Design review of the part built by this model. Coordinates are the model's own, in mm. A direction names the side the tool comes from. Give positions to 0.01 mm unless a question says otherwise; leave off trailing zeros. Order: outer loops, then holes, each group sorted by start corner. A loop starts at its lowest first (then second) coordinate and runs counter-clockwise, first axis right, second up. Notation, with made-up numbers: (9, 44.5) -> (23, 44.5) arc R28 ccw to (23, 80.5) -> close; hole circle Ø10 at (20, 77.5). An arc over 180 degrees is marked (long way). Answer in a Markdown table with one row per item. Add a question column.
```python
from build123d import *

# Parameters (mm, degrees)
CROQUIS1_W                = 13
CROQUIS1_H                = 80
SALIENTE_EXTRUIR1_DEPTH   = 4
CROQUIS1_W_2              = 10
SALIENTE_EXTRUIR1_2_DEPTH = 4
SALIENTE_EXTRUIR1_3_DEPTH = 4
CROQUIS2_W                = 13
CROQUIS2_H                = 13
CROQUIS2_W_2              = 10
CROQUIS2_H_2              = 10
SALIENTE_EXTRUIR2_DEPTH   = 10
CROQUIS3_W                = 13
CROQUIS3_H                = 80
CROQUIS3_W_2              = 10
SALIENTE_EXTRUIR3_DEPTH   = 2.2
CROQUIS4_W                = 80
CROQUIS4_H                = 10
CROQUIS4_H_2              = 13
SALIENTE_EXTRUIR4_DEPTH   = 4
CROQUIS5_W                = 80
CROQUIS5_H                = 80
CROQUIS5_W_2              = 75.6
CROQUIS5_H_2              = 75.6
SALIENTE_EXTRUIR5_DEPTH   = 15
CHAFL_N2_SIZE             = 6.4
CHAFL_N3_SIZE             = 6
CHAFL_N4_SIZE             = 2.2
CROQUIS6_W                = 10
CROQUIS6_H                = 10
CORTAR_EXTRUIR1_DEPTH     = 0.4
REDONDEO1_R               = 1
CHAFL_N1_SIZE             = 1


with BuildPart() as part:
    # Croquis1 → Saliente-Extruir1 (new body)
    with BuildSketch(Plane(origin=(0, 0, 0), x_dir=(0, 1, 0), z_dir=(0, 0, 1))):
        Rectangle(CROQUIS1_W, CROQUIS1_H)
    extrude(amount=SALIENTE_EXTRUIR1_DEPTH)



with BuildPart() as body_2:
    # Croquis1 → Saliente-Extruir1 2 (new body)
    with BuildSketch(Plane(origin=(0, 0, 0), x_dir=(0, 1, 0), z_dir=(0, 0, 1))):
        with Locations((35, 0)):
            Rectangle(CROQUIS1_W_2, CROQUIS1_H)
    extrude(amount=SALIENTE_EXTRUIR1_2_DEPTH)


with BuildPart() as body_3:
    # Croquis1 → Saliente-Extruir1 3 (new body)
    with BuildSketch(Plane(origin=(0, 0, 0), x_dir=(0, 1, 0), z_dir=(0, 0, 1))):
        with Locations((-35, 0)):
            Rectangle(CROQUIS1_W_2, CROQUIS1_H)
    extrude(amount=SALIENTE_EXTRUIR1_3_DEPTH)


with BuildPart() as part_1:
    add(part.part)

    add(body_2.part)  # Saliente-Extruir2 merges body 2

    add(body_3.part)  # Saliente-Extruir2 merges body 3
    # Croquis2 → Saliente-Extruir2 (add)
    with BuildSketch(Plane.XY.offset(4)):
        Rectangle(CROQUIS2_W, CROQUIS2_H)
        with Locations((-35, 0)):
            Rectangle(CROQUIS2_W_2, CROQUIS2_H)
        with Locations((35, 0)):
            Rectangle(CROQUIS2_W_2, CROQUIS2_H)
        with Locations((0, 35)):
            Rectangle(CROQUIS2_W, CROQUIS2_H_2)
        with Locations((-35, 35)):
            Rectangle(CROQUIS2_W_2, CROQUIS2_H_2)
        with Locations((35, 35)):
            Rectangle(CROQUIS2_W_2, CROQUIS2_H_2)
        with Locations((35, -35)):
            Rectangle(CROQUIS2_W_2, CROQUIS2_H_2)
        with Locations((-35, -35)):
            Rectangle(CROQUIS2_W_2, CROQUIS2_H_2)
        with Locations((0, -35)):
            Rectangle(CROQUIS2_W, CROQUIS2_H_2)
    extrude(amount=SALIENTE_EXTRUIR2_DEPTH)

    # Croquis3 → Saliente-Extruir3 (add)
    with BuildSketch(Plane.XY.offset(14)):
        Rectangle(CROQUIS3_W, CROQUIS3_H)
        with Locations((-35, 0)):
            Rectangle(CROQUIS3_W_2, CROQUIS3_H)
        with Locations((35, 0)):
            Rectangle(CROQUIS3_W_2, CROQUIS3_H)
    extrude(amount=-SALIENTE_EXTRUIR3_DEPTH)

    # Croquis4 → Saliente-Extruir4 (add)
    with BuildSketch(Plane.XY.offset(14)):
        with Locations((0, -35)):
            Rectangle(CROQUIS4_W, CROQUIS4_H)
        Rectangle(CROQUIS4_W, CROQUIS4_H_2)
        with Locations((0, 35)):
            Rectangle(CROQUIS4_W, CROQUIS4_H)
        with Locations((0, 16.5)):
            Rectangle(CROQUIS4_W, CROQUIS4_H)
        with Locations((0, -16.5)):
            Rectangle(CROQUIS4_W, CROQUIS4_H)
    extrude(amount=SALIENTE_EXTRUIR4_DEPTH)

    # Croquis5 → Saliente-Extruir5 (add)
    with BuildSketch(Plane.XY.offset(14)):
        Rectangle(CROQUIS5_W, CROQUIS5_H)
        Rectangle(CROQUIS5_W_2, CROQUIS5_H_2, mode=Mode.SUBTRACT)
    extrude(amount=SALIENTE_EXTRUIR5_DEPTH)

    # Chaflán2
    chafl_n2_edges = [part_1.edges().sort_by_distance(p)[0] for p in [
        (0, -30, 11.8),
        (-35, 6.5, 11.8),
        (-35, -6.5, 11.8),
        (-35, 30, 11.8),
        (-35, -30, 11.8),
        (35, 6.5, 11.8),
        (35, 30, 11.8),
        (35, -6.5, 11.8),
        (35, -30, 11.8),
        (0, 6.5, 11.8),
        (0, -6.5, 11.8),
        (0, 30, 11.8),
    ]]
    chamfer(chafl_n2_edges, length=CHAFL_N2_SIZE)

    # Chaflán3
    chafl_n3_edges = [part_1.edges().sort_by_distance(p)[0] for p in [
        (-6.5, -35, 14),
        (30, -35, 14),
        (6.5, 35, 14),
        (-30, 35, 14),
        (6.5, -35, 14),
        (-6.5, 35, 14),
        (-30, -35, 14),
        (30, 35, 14),
    ]]
    chamfer(chafl_n3_edges, length=CHAFL_N3_SIZE)

    # Chaflán4
    chafl_n4_edges = [part_1.edges().sort_by_distance(p)[0] for p in [
        (30, 16.5, 14),
        (30, -16.5, 14),
        (6.5, -16.5, 14),
        (-6.5, -16.5, 14),
        (-30, -16.5, 14),
        (6.5, 16.5, 14),
        (-30, 16.5, 14),
    ]]
    chamfer(chafl_n4_edges, length=CHAFL_N4_SIZE - 0.0001)  # a hair under: the kernel refuses the full size

    # Croquis6 → Cortar-Extruir1 (cut)
    with BuildSketch(Plane(origin=(-40, 0, 0), x_dir=(0, -1, 0), z_dir=(-1, 0, 0))):
        with Locations((0, 14.5)):
            Rectangle(CROQUIS6_W, CROQUIS6_H)
    extrude(amount=-CORTAR_EXTRUIR1_DEPTH, mode=Mode.SUBTRACT)

    # Redondeo1
    redondeo1_edges = [part_1.edges().sort_by_distance(p)[0] for p in [
        (-39.8, -5, 19.5),
        (-39.8, -5, 9.5),
        (-39.8, 5, 9.5),
        (-39.8, 5, 19.5),
    ]]
    fillet(redondeo1_edges, radius=REDONDEO1_R)

    # Chaflán1
    chafl_n1_edges = [part_1.edges().sort_by_distance(p)[0] for p in [
        (-40, 40, 14.5),
        (-40, -40, 14.5),
        (40, -40, 14.5),
        (40, 6.5, 2.7),
        (-40, 6.5, 2.7),
        (-30, 6.5, 4.7),
        (-6.5, 6.5, 4.7),
        (6.5, 6.5, 4.7),
        (30, 6.5, 4.7),
        (6.5, -6.5, 4.7),
        (-30, -6.5, 4.7),
        (-40, -6.5, 2.7),
        (40, -6.5, 2.7),
        (-40, -18.25, 11.8),
        (30, 30, 4.7),
        (-6.5, 30, 4.7),
        (-30, 30, 4.7),
        (-40, 30, 2.7),
        (40, 30, 2.7),
        (-40, 18.25, 11.8),
        (40, -30, 2.7),
        (-40, -30, 2.7),
        (-30, -30, 4.7),
        (6.5, -30, 4.7),
        (30, -30, 4.7),
        (40, 18.25, 11.8),
        (40, -18.25, 11.8),
        (-40, -9.7, 8.6),
        (-40, 26.8, 8.6),
        (-40, 9.7, 8.6),
        (-40, -26.8, 8.6),
        (40, 9.7, 8.6),
        (40, 26.8, 8.6),
        (40, -9.7, 8.6),
        (40, -26.8, 8.6),
        (30, 40, 6),
        (30, -40, 6),
        (-30, 40, 6),
        (-30, -40, 6),
        (6.5, 40, 6),
        (-6.5, -40, 6),
        (6.5, -40, 6),
        (-6.5, 40, 6),
        (40, 40, 14.5),
    ]]
    chamfer(chafl_n1_edges, length=CHAFL_N1_SIZE)


solid = part_1.part
```
1) Add section B-B, the plane z = 22. Write out the cut boundary in (x, y), and give its area (3 significant figures).
2) Clearance check with flat-ended pins moving along their axes: P1, Ø4, axis at x = -5, y = -27.5, coming from the +Z side; P2, Ø8, axis at x = -22, y = 33.5, coming from the +Z side; P3, Ø10, axis at y = 12, z = 11.5, coming from the -X side; P4, Ø8, axis at x = -1.5, y = -16.5, coming from the -Z side. State where each tip first meets the part, or that it passes through.
3) Add section C-C, the plane y = 26. Write out the cut boundary in (x, z), and give its area (3 significant figures).
4) For L1, parallel to X at y = 5.5, z = 11.25; L2, parallel to Y at x = 12, z = 14.5, list the stretches that pass through material, from the lowest coordinate up.
5) Machinability: for faces 4 (the face through (-1, -30, 2)), 5 (the face through (18, 0, 14)), 6 (the face through (39.493, 27.1, 8.998)), 7 (the face through (18, 17, 14)), 8 (the face through (-1, -6.5, 16)), which of the approach directions +Z, -Z, +X, -X, +Y, -Y give a long, thin tool a straight path to every point of the face, cutting with its end or side? Answer none if there is none.
6) Add section A-A, the plane z = 2.5. Write out the cut boundary in (x, y), and give its area (3 significant figures).
7) Mouldability with a two-part tool opening along X and no side actions: class faces 1 (the face through (-35, -18, 11.8)), 2 (the face through (-18, 35, 14)), 3 (the face through (39.493, -27.1, 8.998)) as +X half, -X half, draft (parallel to the pull), parting line (faces both ways), or undercut.
8) Add section D-D, the plane y = -1.5. Write out the cut boundary in (x, z).
Verdict:
| question | item | result |
|---|---|---|
| 1 | outline | (-40, -39) -> (-39, -40) -> (39, -40) -> (40, -39) -> (40, 39) -> (39, 40) -> (-39, 40) -> (-40, 39) -> close; hole (-37.8, -37.8) -> (37.8, -37.8) -> (37.8, 37.8) -> (-37.8, 37.8) -> close |
| 1 | area | 683 mm2 |
| 2 | P1 | stops at z = 14 |
| 2 | P2 | stops at z = 18 |
| 2 | P3 | stops at x = -40 |
| 2 | P4 | stops at z = 11.4 |
| 3 | outline | (-40, 10.81) -> (-39, 9.4) -> (-30, 9.4) -> (-30, 14) -> (-37.8, 14) -> (-37.8, 29) -> (-40, 29) -> close; (-6.5, 9.4) -> (6.5, 9.4) -> (6.5, 14) -> (-6.5, 14) -> close; (30, 9.4) -> (39, 9.4) -> (40, 10.81) -> (40, 29) -> (37.8, 29) -> (37.8, 14) -> (30, 14) -> close |
| 3 | area | 216 mm2 |
| 4 | L1 | x = -40 to -30, -6.5 to 6.5, 30 to 40 |
| 4 | L2 | y = -40 to -30, -21.5 to -11.5, -6.5 to 6.5, 11.5 to 21.5, 30 to 40 |
| 5 | face 4 | -Z, +X, -X |
| 5 | face 5 | none |
| 5 | face 6 | -Z, +X |
| 5 | face 7 | -Z |
| 5 | face 8 | +Z |
| 6 | outline | (-40, -39) -> (-39, -40) -> (39, -40) -> (40, -39) -> (40, -31) -> (39, -30) -> (-39, -30) -> (-40, -31) -> close; (-40, -5.5) -> (-39, -6.5) -> (39, -6.5) -> (40, -5.5) -> (40, 5.5) -> (39, 6.5) -> (-39, 6.5) -> (-40, 5.5) -> close; (-40, 31) -> (-39, 30) -> (39, 30) -> (40, 31) -> (40, 39) -> (39, 40) -> (-39, 40) -> (-40, 39) -> close |
| 6 | area | 2,630 mm2 |
| 7 | face 1 | draft |
| 7 | face 2 | undercut |
| 7 | face 3 | +X half |
| 8 | outline | (-40, 0) -> (40, 0) -> (40, 29) -> (37.8, 29) -> (37.8, 18) -> (-37.8, 18) -> (-37.8, 29) -> (-40, 29) -> (-40, 19.5) -> (-39.6, 19.5) -> (-39.6, 9.5) -> (-40, 9.5) -> close; hole (-30, 4) -> (-6.5, 4) -> (-6.5, 14) -> (-30, 14) -> close; hole (6.5, 4) -> (30, 4) -> (30, 14) -> (6.5, 14) -> close |
